Geometry: final body of the model. Coordinates: model frame, mm. Face numbers are marked on the shaded views. Coordinates: 2 decimals unless noted, no trailing zeros. Loops run counter-clockwise (first coordinate to the right, second up) from the corner with the lowest first, then second, coordinate; pieces in that order, holes last. Notation, with made-up numbers: (-1, 42.25) -> (40, 42.25) arc R25 cw to (40, 77.25) -> close; hole circle Ø4 at (84, 14.25). An arc over 180 degrees is marked (long way). One line per item, written item: value. Start each with the question number.
from build123d import *

# Parameters (mm, degrees)
F1_DEPTH      = 125
F1_DEPTH_BACK = 125
F6_DEPTH      = 5.001
F7_DEPTH      = 5.001
F8_DEPTH      = 2
F9_DEPTH      = 2
F10_DEPTH     = 2
F11_DEPTH     = 2
F12_W         = 30
F12_H         = 40
F13_DEPTH     = 40.001
F14_R         = 17.5


with BuildPart() as f1:
    # F0 (on Front) → F1 (new body, two sides)
    with BuildSketch(Plane.XZ) as f1_sk:
        Polygon((-20, -20), (20, -20), (20, 20), (15, 20), (15, -15), (-15, -15), (-15, 20), (-20, 20), align=None)
    extrude(amount=F1_DEPTH)
    extrude(f1_sk.sketch, amount=-F1_DEPTH_BACK)

    # F3 (on face) → F6 (cut, through all)
    with BuildSketch(Plane(origin=(15, 0, 0), x_dir=(0, -1, 0), z_dir=(-1, 0, 0))):
        with BuildLine():
            Line((107.5, 7.5), (0, 7.5))
            Line((0, 7.5), (-107.5, 7.5))
            ThreePointArc((-107.5, 7.5), (-112.5, 2.5), (-107.5, -2.5))
            Line((-107.5, -2.5), (0, -2.5))
            Line((0, -2.5), (107.5, -2.5))
            ThreePointArc((107.5, -2.5), (112.5, 2.5), (107.5, 7.5))
        make_face()
    extrude(amount=-F6_DEPTH, mode=Mode.SUBTRACT)

    # F2 (on face) → F7 (cut, through all)
    with BuildSketch(Plane.YZ.offset(-15)):
        with BuildLine():
            Line((107.5, 7.5), (0, 7.5))
            Line((0, 7.5), (-107.5, 7.5))
            ThreePointArc((-107.5, 7.5), (-112.5, 2.5), (-107.5, -2.5))
            Line((-107.5, -2.5), (0, -2.5))
            Line((0, -2.5), (107.5, -2.5))
            ThreePointArc((107.5, -2.5), (112.5, 2.5), (107.5, 7.5))
        make_face()
    extrude(amount=-F7_DEPTH, mode=Mode.SUBTRACT)

    # F3 (on face) → F8 (cut)
    with BuildSketch(Plane(origin=(15, 0, 0), x_dir=(0, -1, 0), z_dir=(-1, 0, 0))):
        with BuildLine():
            Line((107.5, 13.75), (0, 13.75))
            Line((0, 13.75), (-107.5, 13.75))
            ThreePointArc((-107.5, 13.75), (-118.75, 2.5), (-107.5, -8.75))
            Line((-107.5, -8.75), (0, -8.75))
            Line((0, -8.75), (107.5, -8.75))
            ThreePointArc((107.5, -8.75), (118.75, 2.5), (107.5, 13.75))
        make_face()
        with BuildLine():
            Line((-107.5, 7.5), (0, 7.5))
            Line((0, 7.5), (107.5, 7.5))
            ThreePointArc((107.5, 7.5), (112.5, 2.5), (107.5, -2.5))
            Line((107.5, -2.5), (0, -2.5))
            Line((0, -2.5), (-107.5, -2.5))
            ThreePointArc((-107.5, -2.5), (-112.5, 2.5), (-107.5, 7.5))
        make_face(mode=Mode.SUBTRACT)
    extrude(amount=-F8_DEPTH, mode=Mode.SUBTRACT)

    # F2 (on face) → F9 (cut)
    with BuildSketch(Plane.YZ.offset(-15)):
        with BuildLine():
            Line((107.5, 13.75), (0, 13.75))
            Line((0, 13.75), (-107.5, 13.75))
            ThreePointArc((-107.5, 13.75), (-118.75, 2.5), (-107.5, -8.75))
            Line((-107.5, -8.75), (0, -8.75))
            Line((0, -8.75), (107.5, -8.75))
            ThreePointArc((107.5, -8.75), (118.75, 2.5), (107.5, 13.75))
        make_face()
        with BuildLine():
            Line((-107.5, 7.5), (0, 7.5))
            Line((0, 7.5), (107.5, 7.5))
            ThreePointArc((107.5, 7.5), (112.5, 2.5), (107.5, -2.5))
            Line((107.5, -2.5), (0, -2.5))
            Line((0, -2.5), (-107.5, -2.5))
            ThreePointArc((-107.5, -2.5), (-112.5, 2.5), (-107.5, 7.5))
        make_face(mode=Mode.SUBTRACT)
    extrude(amount=-F9_DEPTH, mode=Mode.SUBTRACT)

    # F4 (on face) → F10 (cut)
    with BuildSketch(Plane(origin=(-20, 0, 0), x_dir=(0, -1, 0), z_dir=(-1, 0, 0))):
        with BuildLine():
            Line((107.5, 13.75), (0, 13.75))
            Line((0, 13.75), (-107.5, 13.75))
            ThreePointArc((-107.5, 13.75), (-118.75, 2.5), (-107.5, -8.75))
            Line((-107.5, -8.75), (0, -8.75))
            Line((0, -8.75), (107.5, -8.75))
            ThreePointArc((107.5, -8.75), (118.75, 2.5), (107.5, 13.75))
        make_face()
        with BuildLine():
            Line((-107.5, 7.5), (0, 7.5))
            Line((0, 7.5), (107.5, 7.5))
            ThreePointArc((107.5, 7.5), (112.5, 2.5), (107.5, -2.5))
            Line((107.5, -2.5), (0, -2.5))
            Line((0, -2.5), (-107.5, -2.5))
            ThreePointArc((-107.5, -2.5), (-112.5, 2.5), (-107.5, 7.5))
        make_face(mode=Mode.SUBTRACT)
    extrude(amount=-F10_DEPTH, mode=Mode.SUBTRACT)

    # F5 (on face) → F11 (cut)
    with BuildSketch(Plane.YZ.offset(20)):
        with BuildLine():
            Line((107.5, 13.75), (0, 13.75))
            Line((0, 13.75), (-107.5, 13.75))
            ThreePointArc((-107.5, 13.75), (-118.75, 2.5), (-107.5, -8.75))
            Line((-107.5, -8.75), (0, -8.75))
            Line((0, -8.75), (107.5, -8.75))
            ThreePointArc((107.5, -8.75), (118.75, 2.5), (107.5, 13.75))
        make_face()
        with BuildLine():
            Line((-107.5, 7.5), (0, 7.5))
            Line((0, 7.5), (107.5, 7.5))
            ThreePointArc((107.5, 7.5), (112.5, 2.5), (107.5, -2.5))
            Line((107.5, -2.5), (0, -2.5))
            Line((0, -2.5), (-107.5, -2.5))
            ThreePointArc((-107.5, -2.5), (-112.5, 2.5), (-107.5, 7.5))
        make_face(mode=Mode.SUBTRACT)
    extrude(amount=-F11_DEPTH, mode=Mode.SUBTRACT)

    # F12 (on face) → F13 (cut, through all)
    with BuildSketch(Plane(origin=(0, 0, -20), x_dir=(1, 0, 0), z_dir=(0, 0, -1))):
        with Locations((0, -105)):
            Rectangle(F12_W, F12_H)
        with Locations((0, 105)):
            Rectangle(F12_W, F12_H)
    extrude(amount=-F13_DEPTH, mode=Mode.SUBTRACT)

    # F14
    f14_edges = [f1.edges().sort_by_distance(p)[0] for p in [
        (-17.5, 125, -20),
        (17.5, 125, -20),
        (-17.5, 125, 20),
        (17.5, 125, 20),
        (17.5, -125, -20),
        (-17.5, -125, -20),
        (17.5, -125, 20),
        (-17.5, -125, 20),
    ]]
    fillet(f14_edges, radius=F14_R)


solid = f1.part
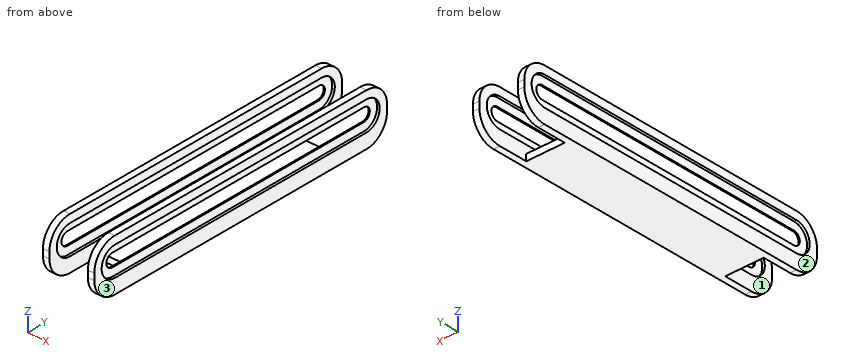
1. Line query: L1, parallel to X at y = 72, z = 9; L2, parallel to X at y = -40.5, z = -12.5; L3, parallel to Z at x = -2, y = 48.5. Output: solid intervals per line, ascending. Write a range as [from, to].
2. Section A-A on y = -76. Count the separate pieces of the cut face and the enclosed holes in it, plus the area to 3 significant figures.
3. Section B-B on z = 10. Return the cut outline in (x, y), plus the area to 3 significant figures.
4. Section C-C on x = -5. Return the cut outline in (y, z).
5. Draft query along X for the marked faces 1, 2 and 3. Return one class per face: released by +X, released by -X, zero draft, split by the parting line, or undercut.
6. Pin query (flat end, axial travel): pin 1 Ø10 at (x, z) = (11, 9.5) entering from -Y; pin 2 Ø1.5 at (x, z) = (-4.5, -17.5) entering from -Y; pin 3 Ø5.5 at (x, z) = (-5, -16.5) entering from +Y; pin 4 Ø3 at (x, y) = (-14, 12) entering from +Z. Return the tip coordinate at first contact, or that it passes through.
Checks:
1. L1: [-18, -17], [17, 18]
1. L2: [-20, -15], [15, 20]
1. L3: [-20, -15]
2. separate pieces: 3
2. enclosed holes: 0
2. area: 350 mm²
3. outline: (-20, -123.31) -> (-15, -123.31) -> (-15, -115.89) -> (-17, -115.89) -> (-17, 115.89) -> (-15, 115.89) -> (-15, 123.31) -> (-20, 123.31) -> (-20, 115.89) -> (-18, 115.89) -> (-18, -115.89) -> (-20, -115.89) -> close; (15, -123.31) -> (20, -123.31) -> (20, -115.89) -> (18, -115.89) -> (18, 115.89) -> (20, 115.89) -> (20, 123.31) -> (15, 123.31) -> (15, 115.89) -> (17, 115.89) -> (17, -115.89) -> (15, -115.89) -> close
3. area: 612 mm²
4. outline: (-85, -20) -> (85, -20) -> (85, -15) -> (-85, -15) -> close
5. face 1: undercut
5. face 2: released by -X
5. face 3: released by +X
6. pin 1: y = -124.54
6. pin 2: y = -85
6. pin 3: y = 85
6. pin 4: z = 20
